The listing builds one solid part. Answer for the finished solid, in the listing's coordinates (mm). A direction names the side the tool comes from. Coordinates: 2 decimals unless noted, no trailing zeros. Write each loop counter-clockwise with the first axis right and the second up, starting at its lowest first coordinate (ties: lowest second). Pieces come first, ordered by that corner, then holes.
```python
from build123d import *

# Parameters (mm, degrees)
SKETCH1_W           = 230
SKETCH1_H           = 90
BOSS_EXTRUDE1_DEPTH = 5
CUT_EXTRUDE1_REACH  = 125.592
SKETCH2_R           = 11
MOVE_FACE2_BY       = 2
SKETCH3_W           = 8.50990482
SKETCH3_H           = 6
CUT_EXTRUDE2_DEPTH  = 10
BOSS_EXTRUDE2_DEPTH = 5
SKETCH6_W           = 30
SKETCH6_H           = 5
BOSS_EXTRUDE3_DEPTH = 5
SKETCH12_W          = 74.296444361
SKETCH12_H          = 104.356394824
CUT_EXTRUDE6_DEPTH  = 10
CUT_EXTRUDE7_DEPTH  = 10
CUT_EXTRUDE8_DEPTH  = 10


with BuildPart() as part:
    # Sketch1 → Boss-Extrude1 (new body)
    with BuildSketch(Plane.XY):
        Rectangle(SKETCH1_W, SKETCH1_H)
    extrude(amount=BOSS_EXTRUDE1_DEPTH)

    # Sketch2 → Cut-Extrude1 (cut, up to next)
    with BuildSketch(Plane.XY.offset(5), mode=Mode.PRIVATE) as cut_extrude1_sk1:
        with Locations((-20.95, 10)):
            Circle(SKETCH2_R)
    cut_extrude1_tool1 = extrude(cut_extrude1_sk1.sketch, amount=-CUT_EXTRUDE1_REACH, mode=Mode.PRIVATE) & part.part
    # Sketch2 → Cut-Extrude1 (cut, up to next)
    with BuildSketch(Plane.XY.offset(5), mode=Mode.PRIVATE) as cut_extrude1_sk2:
        with Locations((20.95, 10)):
            Circle(SKETCH2_R)
    cut_extrude1_tool2 = extrude(cut_extrude1_sk2.sketch, amount=-CUT_EXTRUDE1_REACH, mode=Mode.PRIVATE) & part.part
    add(cut_extrude1_tool1.solids().sort_by_distance((-20.95, 10, 5))[0], mode=Mode.SUBTRACT)
    add(cut_extrude1_tool2.solids().sort_by_distance((20.95, 10, 5))[0], mode=Mode.SUBTRACT)

    # Move Face2: a face moved outward by 2.0
    extrude(part.faces().sort_by_distance((0, 45, 2.5))[0], amount=MOVE_FACE2_BY, dir=(0, 1, 0))

    # Sketch3 → Cut-Extrude2 (cut)
    with BuildSketch(Plane.XY.offset(5)):
        with Locations((-110.74504759, 44)):
            Rectangle(SKETCH3_W, SKETCH3_H)
    extrude(amount=-CUT_EXTRUDE2_DEPTH, mode=Mode.SUBTRACT)

    # Sketch4 → Boss-Extrude2 (add)
    with BuildSketch(Plane.XY.offset(5)):
        with BuildLine():
            Line((-135.913924796, 10.610415662), (-138.38302872, 1.395594371))
            Line((-138.38302872, 1.395594371), (-142.246732025, 2.430870552))
            Line((-142.246732025, 2.430870552), (-146.129017701, -12.058016843))
            Line((-146.129017701, -12.058016843), (-142.265314396, -13.093293023))
            Line((-142.265314396, -13.093293023), (-144.335866757, -20.820699634))
            Line((-144.335866757, -20.820699634), (-138.540311799, -22.373613904))
            Line((-138.540311799, -22.373613904), (-141.646140341, -33.96472382))
            ThreePointArc((-141.646140341, -33.96472382), (-140.955850397, -37.435045716), (-137.782437035, -39))
            Line((-137.782437035, -39), (-125.782437035, -39))
            Line((-125.782437035, -39), (-125.782437035, -45))
            Line((-125.782437035, -45), (-115, -45))
            Line((-115, -45), (-115, 41))
            Line((-115, 41), (-119.257422168, 41))
            ThreePointArc((-119.257422168, 41), (-121.083706455, 40.380060021), (-122.155199647, 38.776457135))
            Line((-122.155199647, 38.776457135), (-122.353798485, 38.03527618))
            Line((-122.353798485, 38.03527618), (-125.459627027, 26.444166265))
            Line((-125.459627027, 26.444166265), (-131.255181984, 27.997080536))
            Line((-131.255181984, 27.997080536), (-133.325734345, 20.269673925))
            Line((-133.325734345, 20.269673925), (-135.913924796, 10.610415662))
        make_face()
    extrude(amount=-BOSS_EXTRUDE2_DEPTH)

    # Sketch6 → Boss-Extrude3 (add)
    with BuildSketch(Plane.XY.offset(5)):
        with Locations((-75.782437035, -47.5)):
            Rectangle(SKETCH6_W, SKETCH6_H)
        with Locations((-5.391218518, -47.5)):
            Rectangle(SKETCH6_W, SKETCH6_H)
        with Locations((65, -47.5)):
            Rectangle(SKETCH6_W, SKETCH6_H)
    extrude(amount=-BOSS_EXTRUDE3_DEPTH)

    # Sketch12 → Cut-Extrude6 (cut)
    with BuildSketch(Plane.XY.offset(5)):
        with Locations((-131.638317361, -5.178197412)):
            Rectangle(SKETCH12_W, SKETCH12_H)
    extrude(amount=-CUT_EXTRUDE6_DEPTH, mode=Mode.SUBTRACT)

    # Sketch13 → Cut-Extrude7 (cut)
    with BuildSketch(Plane.XY.offset(5)):
        Polygon((-38.486827777, -37), (-37.036827777, -37), (-37.036827777, -33.5), (-38.486827777, -33.5), (-38.486827777, -27), (-42.686827777, -27), (-42.686827777, -33.5), (-44.136827777, -33.5), (-44.136827777, -37), (-42.686827777, -37), (-42.686827777, -45), (-38.486827777, -45), align=None)
        Polygon((101.7, -37), (103.15, -37), (103.15, -33.5), (101.7, -33.5), (101.7, -27), (97.5, -27), (97.5, -33.5), (96.05, -33.5), (96.05, -37), (97.5, -37), (97.5, -45), (101.7, -45), align=None)
        Polygon((107, 28.602956743), (107, 30.052956743), (103.5, 30.052956743), (103.5, 28.602956743), (97, 28.602956743), (97, 24.402956743), (103.5, 24.402956743), (103.5, 22.952956743), (107, 22.952956743), (107, 24.402956743), (115, 24.402956743), (115, 28.602956743), align=None)
        Polygon((-66.809520372, 39), (-68.259520372, 39), (-68.259520372, 35.5), (-66.809520372, 35.5), (-66.809520372, 29), (-62.609520372, 29), (-62.609520372, 35.5), (-61.159520372, 35.5), (-61.159520372, 39), (-62.609520372, 39), (-62.609520372, 47), (-66.809520372, 47), align=None)
    extrude(amount=-CUT_EXTRUDE7_DEPTH, mode=Mode.SUBTRACT)

    # Sketch14 → Cut-Extrude8 (cut)
    with BuildSketch(Plane.XY.offset(5)):
        with BuildLine():
            Line((94.447030587, -16.995566986), (59.447030587, -16.043949671))
            ThreePointArc((59.447030587, -16.043949671), (47.777611866, -3.722234421), (60.099327116, 7.947184301))
            Line((60.099327116, 7.947184301), (95.099327116, 6.995566986))
            ThreePointArc((95.099327116, 6.995566986), (106.768745837, -5.326148264), (94.447030587, -16.995566986))
        make_face()
    extrude(amount=-CUT_EXTRUDE8_DEPTH, mode=Mode.SUBTRACT)


solid = part.part
```
(1) For a pull along Y with two mould halves and no side action, classify faces 6 (the flat face through (9, -1, 0)), 7 (the flat face through (-41, -27, 3)), 8 (the flat face through (96.05, -35, 3)), 9 (the cylindrical face through (106.773, -5.062, 2.535)) as pulls with the +Y half, pulls with the -Y half, needs draft (parallel to the pull), parting line crosses it, or undercut.
(2) Each of these flat-tipped pins is pushed along its axis until it touches: pin 1 (1.2 mm diameter, centred on x = 97, z = 1.5, fed in from -Y); pin 2 (13 mm diameter, centred on x = -20.95, y = 10, fed in from +Z); pin 3 (2 mm diameter, centred on y = 27, z = 3.5, fed in from +X). Where does it stop, or does it pass through?
(3) Section C-C, the plane z = 2.6 is taken. State how many separate pieces and enclosed holes the cut face has, plus the area to 3 significant figures.
(4) Section A-A, the plane y = 10 is taken. Write down the section's boundary in (x, z), plus the area to 3 significant figures.
(5) Find the intervals of material crossed by probe 1 along X at (y, z) = (10.5, 4.15); probe 2 along X at (y, z) = (-31.5, 4.2); probe 3 along X at (y, z) = (34.5, 2.85), in increasing order.
(6) Section B-B, the plane x = -29.5 is taken. Write down the section's boundary in (y, z).
(7) Which of the six approach directions +Z, -Z, +X, -X, +Y, -Y give full straight-line access (tool end or side, diameter ignored) to faces 1 (the flat face through (97, 27, 3)), 2 (the flat face through (-52, -45, 3)), 3 (the flat face through (105, 30.053, 3)), 4 (the flat face through (89, -45, 3)), 5 (the flat face through (-66.81, 32, 3))?
(8) Section D-D, the plane x = 99.5 is taken. Write down the section's boundary in (y, z).
Solution:
1. face 6: needs draft
1. face 7: pulls with the -Y half
1. face 8: undercut
1. face 9: undercut
2. pin 1: stops at y = -45
2. pin 2: passes through
2. pin 3: stops at x = 97
3. separate pieces: 1
3. enclosed holes: 3
3. area: 17,300 mm2
4. outline: (-94.49, 0) - (-31.95, 0) - (-31.95, 5) - (-94.49, 5) - close; (-9.95, 0) - (9.95, 0) - (9.95, 5) - (-9.95, 5) - close; (31.95, 0) - (115, 0) - (115, 5) - (31.95, 5) - close
4. area: 827 mm2
5. probe 1: x = -94.49 to -31.94, -9.96 to 9.96, 31.94 to 115
5. probe 2: x = -94.49 to -42.69, -38.49 to 97.5, 101.7 to 115
5. probe 3: x = -94.49 to -66.81, -62.61 to 115
6. outline: (-45, 0) - (3.08, 0) - (3.08, 5) - (-45, 5) - close; (16.92, 0) - (47, 0) - (47, 5) - (16.92, 5) - close
7. face 1: +Z, -Z, +X
7. face 2: +Z, -Z, -Y
7. face 3: +Z, -Z
7. face 4: +Z, -Z, +X, -Y
7. face 5: +Z, -Z, +Y
8. outline: (-27, 0) - (-16.03, 0) - (-16.03, 5) - (-27, 5) - close; (6.03, 0) - (24.4, 0) - (24.4, 5) - (6.03, 5) - close; (28.6, 0) - (47, 0) - (47, 5) - (28.6, 5) - close
